```python
from build123d import *

# Parameters (mm, degrees)
F2_R     = 11.382986
F3_DEPTH = 25
F4_SIZE  = 0.5
F5_SIZE  = 0.5
F6_SIZE  = 0.5


with BuildPart() as f1:
    # F0 (on Front) → F1 (revolve)
    with BuildSketch(Plane.XZ):
        Polygon((0, 10), (0, 0), (31, 0), (31, 3), (21, 3), (21, 4), (3, 4), (3, 10), align=None)
    revolve(axis=Axis((15.5, 0, 0), (1, 0, 0)))

    # F2 (on face) → F3 (cut)
    with BuildSketch(Plane(origin=(0, 0, 0), x_dir=(0, -1, 0), z_dir=(-1, 0, 0))):
        Circle(F2_R)
        Polygon((-5.463653, 7.787273), (4.01215, 8.625299), (9.475803, 0.838026), (5.463653, -7.787273), (-4.01215, -8.625299), (-9.475803, -0.838026), align=None, mode=Mode.SUBTRACT)
    extrude(amount=-F3_DEPTH, mode=Mode.SUBTRACT)

    # F4
    f4_edges = [f1.edges().sort_by_distance(p)[0] for p in [
        (21, 0, -4),
    ]]
    chamfer(f4_edges, length=F4_SIZE)

    # F5
    f5_edges = [f1.edges().sort_by_distance(p)[0] for p in [
        (31, 0, -3),
    ]]
    chamfer(f5_edges, length=F5_SIZE)

    # F6
    f6_edges = [f1.edges().sort_by_distance(p)[0] for p in [
        (0, 6.743976, -4.731663),
        (0, -0.725752, -8.206286),
        (0, -7.469728, -3.474624),
        (0, -6.743976, 4.731663),
        (0, 0.725752, 8.206286),
        (0, 7.469728, 3.474624),
    ]]
    chamfer(f6_edges, length=F6_SIZE)


solid = f1.part
```
Verification items for the finished model (mm, model axes). A direction names the side the tool comes from. Round coordinates to 2 decimals unless told otherwise and drop trailing zeros. Write each loop counter-clockwise with the first axis right and the second up, starting at its lowest first coordinate (ties: lowest second). Pieces come first, ordered by that corner, then holes. Notation, with made-up numbers: (51, 9.25) - (72, 9.25) arc R7 ccw to (72, 19.25) - close; hole circle Ø10 at (84.5, -28). An arc over 180 degrees is marked (long way). Answer as a JSON object with one key per item and string values. Group by question number.
Q1. Go/stop test with flat-tipped pins: pin 1 Ø10 at (x, y) = (7.5, 5) entering from +Z; pin 2 Ø1.5 at (x, z) = (10.5, 2) entering from +Y; pin 3 Ø1.5 at (x, z) = (20.5, 0) entering from +Y. Record where each tip stops, or that it passes through.
Q2. Section check D-D, the plane z = 0. Enter the section's corners in (x, y).
Q3. Section check B-B, the plane z = 6.25. Enter the section's corners in (x, y).
Q4. Thickness scan on line 1 (X direction, y = -3, z = -0.5); line 2 (X direction, y = 3.25, z = -6.75); line 3 (Z direction, x = 23, y = -2.5). Record the ranges inside material, lowest first.
Q5. Section check C-C, the plane x = 22.5. Enter the section's corners in (y, z).
Q6. Tool access check on faces 1 (the cylindrical face through (26, 0, -3)), 2 (the flat face through (1.732, 6.706, -4.786)). Record the directions out of +Z, -Z, +X, -X, +Y, -Y that give a thin tool (end or side, any length) a straight path to the whole face; none if there is none.
Q7. Section check A-A, the plane y = 0. Enter the section's corners in (x, z).
Found:
{
 "1": {"pin 1": "stops at z = 8.02", "pin 2": "stops at y = 3.8", "pin 3": "stops at y = 4"},
 "2": {"outline": "(0, -8.53) - (0.5, -9.09) - (3, -9.09) - (3, -4) - (20.5, -4) - (21, -3.5) - (21, -3) - (30.5, -3) - (31, -2.5) - (31, 2.5) - (30.5, 3) - (21, 3) - (21, 3.5) - (20.5, 4) - (3, 4) - (3, 9.09) - (0.5, 9.09) - (0, 8.53) - close"},
 "3": {"outline": "(0, -5.07) - (0.5, -5.68) - (3, -5.68) - (3, 6.18) - (0.5, 6.18) - (0, 5.63) - close"},
 "4": {"line 1": "x = 0 to 21", "line 2": "x = 0 to 3", "line 3": "z = -1.66 to 1.66"},
 "5": {"outline": "circle Ø6 at (0, 0)"},
 "6": {"face 1": "+X", "face 2": "-Z, +X, -X, +Y"},
 "7": {"outline": "(0, -7.77) - (0.5, -8.27) - (3, -8.27) - (3, -4) - (20.5, -4) - (21, -3.5) - (21, -3) - (30.5, -3) - (31, -2.5) - (31, 2.5) - (30.5, 3) - (21, 3) - (21, 3.5) - (20.5, 4) - (3, 4) - (3, 8.27) - (0.5, 8.27) - (0, 7.77) - close"}
}
